Part model, mm, in its own coordinate system. A direction names the side the tool comes from. Give positions to 0.01 mm unless a question says otherwise; leave off trailing zeros. Order: outer loops, then holes, each group sorted by start corner. A loop starts at its lowest first (then second) coordinate and runs counter-clockwise, first axis right, second up. Notation, with made-up numbers: M 46,82 L 82,82 A5 cw 82,86 Z; hole C 82.25,-1.75 d8. An arc over 180 degrees is marked long. Answer as a JSON object with one key per item and string values.
from build123d import *

# Parameters (mm, degrees)
SKETCH2_R = 1


with BuildPart() as part:
    # Sweep1: sweep along a path in Sketch1
    with BuildLine(Plane.XY) as sweep1_path:
        Line((-17.55, 78), (-7.5, 78))
        ThreePointArc((-7.5, 78), (-6.439339828, 77.560660172), (-6, 76.5))
        Line((-6, 76.5), (-6, 1.5))
        ThreePointArc((-6, 1.5), (-5.560660172, 0.439339828), (-4.5, 0))
        Line((-4.5, 0), (-3.5, 0))
        Line((-3.5, 0), (0, 0))
    # Sketch2 → Sweep1 (sweep)
    with BuildSketch(Plane(origin=(0, 0, 0), x_dir=(0, 0, -1), z_dir=(1, 0, 0))):
        Circle(SKETCH2_R)
    sweep(path=sweep1_path.line)


solid = part.part
1. Cut at B-B on y = 64. Give the cut face in (x, z), plus the area to 3 significant figures.
Worked answers:
{"outline": "C -6,0 d2", "area": "3.14 mm^2"}
2. Cut at A-A on z = -0.6. Give the cut face in (x, y), plus the area to 3 significant figures.
Worked answers:
{"outline": "M -17.55,77.2 L -7.5,77.2 A0.7 cw -6.8,76.5 L -6.8,1.5 A2.3 ccw -4.5,-0.8 L 0,-0.8 L 0,0.8 L -4.5,0.8 A0.7 cw -5.2,1.5 L -5.2,76.5 A2.3 ccw -7.5,78.8 L -17.55,78.8 Z", "area": "151 mm^2"}
3. Probe line 1 along Y through (x, z) = (-15.25, 0); line 2 along X through (y, z) = (42.5, -0.05); line 3 along X through (y, z) = (63.5, 0.8). List the from-to ranges inside material, lowest first.
Worked answers:
{"line 1": "y = 77 to 79", "line 2": "x = -7 to -5", "line 3": "x = -6.6 to -5.4"}
4. Which spindle directions (+Z, -Z, +X, -X, +Y, -Y) get a long thin tool onto all of the face, cutting with end or side? Do faces 1 (the cylindrical face through (-5, 38, 0)), 2 (the cylindrical face through (-2, -1, 0)), 3 (the cylindrical face through (-12, 77, 0)). Say none if no direction does.
Worked answers:
{"face 1": "none", "face 2": "+X", "face 3": "-X"}
5. Cut at C-C on x = -1.5. Give the cut face in (y, z).
Worked answers:
{"outline": "C 0,0 d2"}
